```python
from build123d import *

# Parameters (mm, degrees)
F1_DEPTH = 101.6
F2_W     = 7.62
F2_H     = 7.62
F3_DEPTH = 22.86


with BuildPart() as f1:
    # F0 (on Front) → F1 (new body)
    with BuildSketch(Plane.XZ):
        Polygon((50.8, 0), (0, 0), (-50.8, 0), (-50.8, -25.4), (50.8, -25.4), align=None)
    extrude(amount=F1_DEPTH)

    # F2 (on face) → F3 (cut)
    with BuildSketch(Plane.XY):
        with Locations((-38.1, -12.7)):
            Rectangle(F2_W, F2_H)
        with Locations((-12.7, -12.7)):
            Rectangle(F2_W, F2_H)
        with Locations((12.7, -12.7)):
            Rectangle(F2_W, F2_H)
        with Locations((38.1, -12.7)):
            Rectangle(F2_W, F2_H)
        with Locations((-38.1, -38.1)):
            Rectangle(F2_W, F2_H)
        with Locations((-12.7, -38.1)):
            Rectangle(F2_W, F2_H)
        with Locations((-38.1, -63.5)):
            Rectangle(F2_W, F2_H)
        with Locations((-38.1, -88.9)):
            Rectangle(F2_W, F2_H)
        with Locations((-12.7, -88.9)):
            Rectangle(F2_W, F2_H)
        with Locations((12.7, -88.9)):
            Rectangle(F2_W, F2_H)
        with Locations((38.1, -88.9)):
            Rectangle(F2_W, F2_H)
        with Locations((38.1, -63.5)):
            Rectangle(F2_W, F2_H)
        with Locations((12.7, -63.5)):
            Rectangle(F2_W, F2_H)
        with Locations((-12.7, -63.5)):
            Rectangle(F2_W, F2_H)
        with Locations((12.7, -38.1)):
            Rectangle(F2_W, F2_H)
        with Locations((38.1, -38.1)):
            Rectangle(F2_W, F2_H)
    extrude(amount=-F3_DEPTH, mode=Mode.SUBTRACT)


solid = f1.part
```
Build history of the part. All positions in model axes, mm. A direction names the side the tool comes from. Coordinates: 2 decimals unless noted, no trailing zeros. Order: outer loops, then holes, each group sorted by start corner. A loop starts at its lowest first (then second) coordinate and runs counter-clockwise, first axis right, second up. Notation, with made-up numbers: (-33, -32.75) -> (19, -32.75) arc R26 ccw to (19, -17.75) -> close; hole circle Ø1 at (0, 61.5). An arc over 180 degrees is marked (long way). Answer in a Markdown table with one row per item. Add a question column.
Q1. Which spindle directions (+Z, -Z, +X, -X, +Y, -Y) get a long thin tool onto all of the face, cutting with end or side? Do faces 5 (the face through (-50.8, -50, -13)), 6 (the face through (-34.29, -64, -11)). Say none if no direction does.
Q2. Mould opens along Y. For faces 1 (the face through (-1, -101.6, -13)), 2 (the face through (38, -89, -22.86)), 3 (the face through (13, -34.29, -11)), 4 (the face through (1, -50, 0)) say: +Y half, -Y half, draft (parallel to the pull), parting line (faces both ways), or undercut.
Q3. Band-saw the part on A-A, the plane x = -11. List the corners of the cut face in (y, z).
Q4. Drop a flat-ended pin along its axis: pin 1 (4 mm diameter, centred on x = -39, y = -64.5, fed in from +Z). Give the stop position or say it passes through.
Q5. Band-saw the part on C-C, the plane z = -3.5. Give the number of separate pieces and of enclosed holes in the cut face, then the cut area to 3 significant figures.
Q6. Band-saw the part on B-B, the plane y = -10.5. List the corners of the cut face in (x, z), then the cut area to 3 significant figures.
Q7. Wall check: line 1 along X through (y, z) = (-40, -19); line 2 along Y through (x, z) = (37.5, -6.5); line 3 along Z through (x, y) = (40.5, -12.5). Give the ranges that are in metal, low to high. Write a range as [from, to].
Answers follow:
| question | item | result |
|---|---|---|
| 1 | face 5 | +Z, -Z, -X, +Y, -Y |
| 1 | face 6 | +Z |
| 2 | face 1 | -Y half |
| 2 | face 2 | undercut |
| 2 | face 3 | undercut |
| 2 | face 4 | draft |
| 3 | outline | (-101.6, -25.4) -> (0, -25.4) -> (0, 0) -> (-8.89, 0) -> (-8.89, -22.86) -> (-16.51, -22.86) -> (-16.51, 0) -> (-34.29, 0) -> (-34.29, -22.86) -> (-41.91, -22.86) -> (-41.91, 0) -> (-59.69, 0) -> (-59.69, -22.86) -> (-67.31, -22.86) -> (-67.31, 0) -> (-85.09, 0) -> (-85.09, -22.86) -> (-92.71, -22.86) -> (-92.71, 0) -> (-101.6, 0) -> close |
| 4 | pin 1 | z = -22.86 |
| 5 | separate pieces | 1 |
| 5 | enclosed holes | 16 |
| 5 | area | 9,390 mm^2 |
| 6 | outline | (-50.8, -25.4) -> (50.8, -25.4) -> (50.8, 0) -> (41.91, 0) -> (41.91, -22.86) -> (34.29, -22.86) -> (34.29, 0) -> (16.51, 0) -> (16.51, -22.86) -> (8.89, -22.86) -> (8.89, 0) -> (-8.89, 0) -> (-8.89, -22.86) -> (-16.51, -22.86) -> (-16.51, 0) -> (-34.29, 0) -> (-34.29, -22.86) -> (-41.91, -22.86) -> (-41.91, 0) -> (-50.8, 0) -> close |
| 6 | area | 1,880 mm^2 |
| 7 | line 1 | [-50.8, -41.91], [-34.29, -16.51], [-8.89, 8.89], [16.51, 34.29], [41.91, 50.8] |
| 7 | line 2 | [-101.6, -92.71], [-85.09, -67.31], [-59.69, -41.91], [-34.29, -16.51], [-8.89, 0] |
| 7 | line 3 | [-25.4, -22.86] |
